CAD build for the part. Positions are in the model's coordinates, mm. A direction names the side the tool comes from. Round coordinates to 2 decimals unless told otherwise and drop trailing zeros. Order: outer loops, then holes, each group sorted by start corner. A loop starts at its lowest first (then second) coordinate and runs counter-clockwise, first axis right, second up.
```python
from build123d import *

# Parameters (mm, degrees)
SKETCH2_R           = 3
BOSS_EXTRUDE1_DEPTH = 60
CUT_EXTRUDE1_DEPTH  = 20


with BuildPart() as part:
    # Sketch2 → Boss-Extrude1 (new body)
    with BuildSketch(Plane.XY):
        with BuildLine():
            Line((-6, 0), (-6, 25))
            Line((-6, 25), (-3, 25))
            Line((-3, 25), (-3, 5.196152423))
            ThreePointArc((-3, 5.196152423), (5.196152423, -3), (-6, 0))
        make_face()
        Circle(SKETCH2_R, mode=Mode.SUBTRACT)
    extrude(amount=BOSS_EXTRUDE1_DEPTH)

    # Sketch3 → Cut-Extrude1 (cut)
    with BuildSketch(Plane.XY.offset(20)):
        with BuildLine():
            Line((-3, 5.196152423), (-6, 5.196152423))
            Line((-6, 5.196152423), (-6, 0))
            ThreePointArc((-6, 0), (5.196152423, -3), (-3, 5.196152423))
        make_face()
    extrude(amount=CUT_EXTRUDE1_DEPTH, mode=Mode.SUBTRACT)


solid = part.part
```
1. Tool access for faces 1 (the face through (-4, 5.196, 30)), 2 (the face through (-4, 6, 60)): list every direction of +Z, -Z, +X, -X, +Y, -Y with a clear straight run to the whole face (end or side of a thin tool).
2. Cut at B-B, the plane y = 4.5. Write the cut outline in (x, z).
3. Cut at D-D, the plane z = 17.5. Write the cut outline in (x, y).
4. Cut at C-C, the plane x = 5.25. Write the cut outline in (y, z), and give its area (3 significant figures).
5. Mould opens along X. For faces 3 (the face through (-3, 0, 50)), 4 (the face through (-5, 25, 30)), 5 (the face through (-6, 12, 30)) say: released by +X, released by -X, zero draft, split by the parting line, or undercut.
6. Cut at A-A, the plane x = 0. Write the cut outline in (y, z).
7. Drill centre lines: line 1 (Z direction, x = -3.5, y = 3); line 2 (Y direction, x = 0, z = 51.5); line 3 (X direction, y = 16, z = 17). Where is each one in solid material? Low to high.
8. Pin check, flat tips, straight feed: P1, Ø4, axis at x = -4, z = 15.5, coming from the -Y side; P2, Ø3, axis at y = 5, z = 9, coming from the +X side; P3, Ø3, axis at x = -4.5, y = 6, coming from the -Z side; P4, Ø1, axis at x = 3.5, z = 14, coming from the +Y side. Stop position of each tip, or through.
Outcome:
1. face 1: +X, -X, -Y
1. face 2: +Z, +X, -X, +Y, -Y
2. outline: (-6, 0) - (3.97, 0) - (3.97, 20) - (-6, 20) - close; (-6, 40) - (3.97, 40) - (3.97, 60) - (-6, 60) - close
3. outline: (-6, 0) arc R6 ccw (long way) to (-3, 5.2) - (-3, 25) - (-6, 25) - close; hole circle Ø6 at (0, 0)
4. outline: (-2.9, 0) - (2.9, 0) - (2.9, 20) - (-2.9, 20) - close; (-2.9, 40) - (2.9, 40) - (2.9, 60) - (-2.9, 60) - close
4. area: 232 mm2
5. face 3: undercut
5. face 4: zero draft
5. face 5: released by -X
6. outline: (-6, 0) - (-3, 0) - (-3, 20) - (-6, 20) - close; (-6, 40) - (-3, 40) - (-3, 60) - (-6, 60) - close; (3, 0) - (6, 0) - (6, 20) - (3, 20) - close; (3, 40) - (6, 40) - (6, 60) - (3, 60) - close
7. line 1: z = 0 to 20, 40 to 60
7. line 2: y = -6 to -3, 3 to 6
7. line 3: x = -6 to -3
8. P1: stops at y = -5.66
8. P2: stops at x = 4.87
8. P3: stops at z = 0
8. P4: stops at y = 5.2
